```python
from build123d import *

# Parameters (mm, degrees)
SKETCH1_R           = 2.5
BOSS_EXTRUDE1_DEPTH = 330


with BuildPart() as part:
    # Sketch1 → Boss-Extrude1 (new body)
    with BuildSketch(Plane(origin=(0, 0, 0), x_dir=(0, 0, -1), z_dir=(1, 0, 0))):
        with BuildLine():
            Line((-4.1, 10), (-8, 10))
            ThreePointArc((-8, 10), (-9.414213562, 9.414213562), (-10, 8))
            Line((-10, 8), (-10, 4.1))
            Line((-10, 4.1), (-9, 3.1))
            Line((-9, 3.1), (-8, 3.1))
            Line((-8, 3.1), (-8, 5))
            Line((-8, 5), (-7.242640687, 5))
            ThreePointArc((-7.242640687, 5), (-6.477273822, 4.847759065), (-5.828427125, 4.414213562))
            Line((-5.828427125, 4.414213562), (-4.537854624, 3.123641061))
            ThreePointArc((-4.537854624, 3.123641061), (-4.104309121, 2.474794364), (-3.952068186, 1.709427499))
            Line((-3.952068186, 1.709427499), (-3.952068186, -1.709427499))
            ThreePointArc((-3.952068186, -1.709427499), (-4.104309121, -2.474794364), (-4.537854624, -3.123641061))
            Line((-4.537854624, -3.123641061), (-5.828427125, -4.414213562))
            ThreePointArc((-5.828427125, -4.414213562), (-6.477273822, -4.847759065), (-7.242640687, -5))
            Line((-7.242640687, -5), (-8, -5))
            Line((-8, -5), (-8, -3.1))
            Line((-8, -3.1), (-9, -3.1))
            Line((-9, -3.1), (-10, -4.1))
            Line((-10, -4.1), (-10, -8))
            ThreePointArc((-10, -8), (-9.414213562, -9.414213562), (-8, -10))
            Line((-8, -10), (-4.1, -10))
            Line((-4.1, -10), (-3.1, -9))
            Line((-3.1, -9), (-3.1, -8))
            Line((-3.1, -8), (-5, -8))
            Line((-5, -8), (-5, -7.242640687))
            ThreePointArc((-5, -7.242640687), (-4.847759065, -6.477273822), (-4.414213562, -5.828427125))
            Line((-4.414213562, -5.828427125), (-3.123641061, -4.537854624))
            ThreePointArc((-3.123641061, -4.537854624), (-2.474794364, -4.104309121), (-1.709427499, -3.952068186))
            Line((-1.709427499, -3.952068186), (1.709427499, -3.952068186))
            ThreePointArc((1.709427499, -3.952068186), (2.474794364, -4.104309121), (3.123641061, -4.537854624))
            Line((3.123641061, -4.537854624), (4.414213562, -5.828427125))
            ThreePointArc((4.414213562, -5.828427125), (4.847759065, -6.477273822), (5, -7.242640687))
            Line((5, -7.242640687), (5, -8))
            Line((5, -8), (3.1, -8))
            Line((3.1, -8), (3.1, -9))
            Line((3.1, -9), (4.1, -10))
            Line((4.1, -10), (8, -10))
            ThreePointArc((8, -10), (9.414213562, -9.414213562), (10, -8))
            Line((10, -8), (10, -4.1))
            Line((10, -4.1), (9, -3.1))
            Line((9, -3.1), (8, -3.1))
            Line((8, -3.1), (8, -5))
            Line((8, -5), (7.242640687, -5))
            ThreePointArc((7.242640687, -5), (6.477273822, -4.847759065), (5.828427125, -4.414213562))
            Line((5.828427125, -4.414213562), (4.537854624, -3.123641061))
            ThreePointArc((4.537854624, -3.123641061), (4.104309121, -2.474794364), (3.952068186, -1.709427499))
            Line((3.952068186, -1.709427499), (3.952068186, 1.709427499))
            ThreePointArc((3.952068186, 1.709427499), (4.104309121, 2.474794364), (4.537854624, 3.123641061))
            Line((4.537854624, 3.123641061), (5.828427125, 4.414213562))
            ThreePointArc((5.828427125, 4.414213562), (6.477273822, 4.847759065), (7.242640687, 5))
            Line((7.242640687, 5), (8, 5))
            Line((8, 5), (8, 3.1))
            Line((8, 3.1), (9, 3.1))
            Line((9, 3.1), (10, 4.1))
            Line((10, 4.1), (10, 8))
            ThreePointArc((10, 8), (9.414213562, 9.414213562), (8, 10))
            Line((8, 10), (4.1, 10))
            Line((4.1, 10), (3.1, 9))
            Line((3.1, 9), (3.1, 8))
            Line((3.1, 8), (5, 8))
            Line((5, 8), (5, 7.242640687))
            ThreePointArc((5, 7.242640687), (4.847759065, 6.477273822), (4.414213562, 5.828427125))
            Line((4.414213562, 5.828427125), (3.123641061, 4.537854624))
            ThreePointArc((3.123641061, 4.537854624), (2.474794364, 4.104309121), (1.709427499, 3.952068186))
            Line((1.709427499, 3.952068186), (-1.709427499, 3.952068186))
            ThreePointArc((-1.709427499, 3.952068186), (-2.474794364, 4.104309121), (-3.123641061, 4.537854624))
            Line((-3.123641061, 4.537854624), (-4.414213562, 5.828427125))
            ThreePointArc((-4.414213562, 5.828427125), (-4.847759065, 6.477273822), (-5, 7.242640687))
            Line((-5, 7.242640687), (-5, 8))
            Line((-5, 8), (-3.1, 8))
            Line((-3.1, 8), (-3.1, 9))
            Line((-3.1, 9), (-4.1, 10))
        make_face()
        Circle(SKETCH1_R, mode=Mode.SUBTRACT)
    extrude(amount=BOSS_EXTRUDE1_DEPTH)


solid = part.part
```
The listing builds one solid part. Answer for the finished solid, in the listing's coordinates (mm). Give positions to 0.01 mm unless a question says otherwise; leave off trailing zeros. Use one line per item in the form item = value. Start each with the question number.
(1) Flat-ended cylindrical pins translate along their axes: pin 1 Ø5 at (y, z) = (-4, 4) entering from -X; pin 2 Ø4 at (x, y) = (141.5, -1) entering from +Z; pin 3 Ø5 at (x, y) = (64, 1) entering from -Z; pin 4 Ø1 at (x, z) = (229, 1) entering from +Y. Find the tip coordinate at first contact, or state that the pin passes through.
(2) The mould has two halves that part along Z. Classify faces 1 (the cylindrical face through (162.69, -2.44, 0.54)), 2 (the flat face through (330, 2, -2)): released by +Z, released by -Z, zero draft, split by the parting line, or undercut.
(3) Consider line 1 (Y direction, x = 29.5, z = 6); line 2 (Y direction, x = 38, z = -7.5); line 3 (Y direction, x = 170.5, z = -4.5). Determine where each line is inside the solid, lowest interval first. Write a range as from..to.
Ans:
q1.pin_1 = 0
q1.pin_2 = 4.42
q1.pin_3 = -9.4
q1.pin_4 = 3.95
q2.face_1 = undercut
q2.face_2 = zero draft
q3.line_1 = -10..-4.57, 4.57..10
q3.line_2 = -10..-5, 5..10
q3.line_3 = -10..-8, -5.92..-3.08, 3.08..5.92, 8..10
